Answer from the drawing. Dimensions are ordinates in mm from the lowest x, y and z of the part. Give positions to 0.01 mm unless a question says otherwise; leave off trailing zeros. Write each loop counter-clockwise with the first axis right and the second up, starting at its lowest first coordinate (ties: lowest second). Pieces come first, ordered by that corner, then holes.
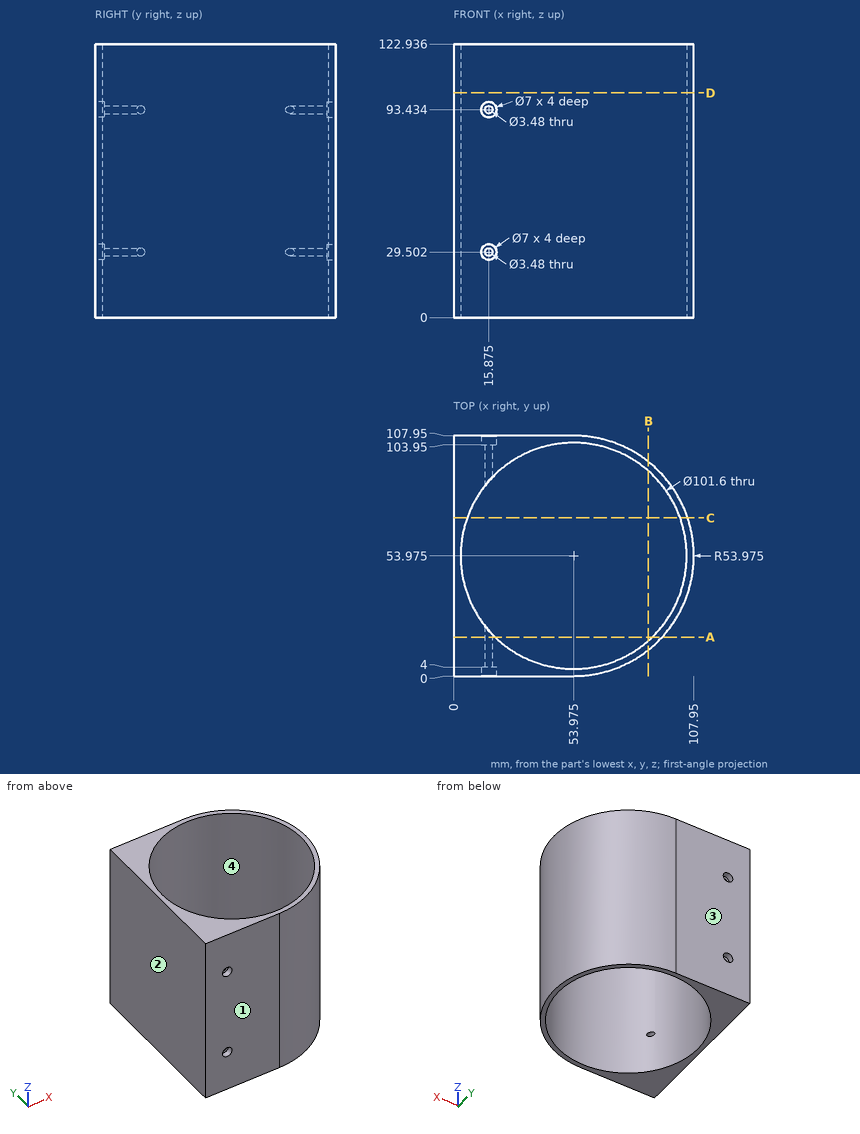
Item 1: Section B-B (x = 87.5) is taken. Write down the section's boundary in (y, z), and give its area (3 significant figures).
Result set:
outline: (11.67, 0) - (15.81, 0) - (15.81, 122.94) - (11.67, 122.94) - close; (92.14, 0) - (96.28, 0) - (96.28, 122.94) - (92.14, 122.94) - close
area: 1,020 mm2
Item 2: Section A-A (y = 17.5) is taken. Write down the section's boundary in (x, z) (1 decimal), and give its area (3 significant figures).
Result set:
outline: (0, 0) - (18.6, 0) - (18.6, 122.9) - (0, 122.9) - close; (89.3, 0) - (93.8, 0) - (93.8, 122.9) - (89.3, 122.9) - close; hole circle Ø3.5 at (15.9, 29.5); hole circle Ø3.5 at (15.9, 93.4)
area: 2,810 mm2
Item 3: Each of these flat-tipped pins is pushed along its axis until it touches: pin 1 Ø5.5 at (x, z) = (15.5, 93) entering from +Y; pin 2 Ø5.5 at (x, z) = (17.5, 31) entering from +Y; pin 3 Ø2 at (x, z) = (15.88, 29.5) entering from +Y; pin 4 Ø4.5 at (x, z) = (15.88, 29.5) entering from -Y. Where does it stop, or does it pass through?
Result set:
pin 1: stops at y = 103.95
pin 2: stops at y = 107.95
pin 3: passes through
pin 4: stops at y = 4
Item 4: Section D-D (z = 101) is taken. Write down the section's boundary in (x, y) (3 decimals).
Result set:
outline: (0, 0) - (53.975, 0) arc R53.975 ccw to (53.975, 107.95) - (0, 107.95) - close; hole circle Ø101.6 at (53.975, 53.975)
Item 5: Find the intervals of material crossed by line 1 along X through (y, z) = (61, 11.5); line 2 along X through (y, z) = (94.5, 8) (1 decimal); line 3 along Y through (x, z) = (24.5, 36), in increasing order.
Result set:
line 1: x = 0 to 3.66, 104.29 to 107.49
line 2: x = 0 to 23.3, 84.6 to 89.6
line 3: y = 0 to 12.6, 95.35 to 107.95
Item 6: Section C-C (y = 71) is taken. Write down the section's boundary in (x, z) (1 decimal), and give its area (3 significant figures).
Result set:
outline: (0, 0) - (6.1, 0) - (6.1, 122.9) - (0, 122.9) - close; (101.8, 0) - (105.2, 0) - (105.2, 122.9) - (101.8, 122.9) - close
area: 1,160 mm2
Item 7: Determine the mould class of the marked faces 1, 2, 3 and 4 for opening direction Y: pulls with the +Y half, pulls with the -Y half, needs draft (parallel to the pull), parting line crosses it, or undercut.
Result set:
face 1: pulls with the -Y half
face 2: needs draft
face 3: pulls with the +Y half
face 4: undercut
